from build123d import *

# Parameters (mm, degrees)
F0_R     = 32
F0_W     = 2
F0_H     = 2
F1_DEPTH = 7
F2_R     = 2.5
F4_R     = 2
F5_DEPTH = 7


with BuildPart() as f1:
    # F0 (on Top) → F1 (new body)
    with BuildSketch(Plane.XY):
        Circle(F0_R)
        with BuildLine():
            ThreePointArc((1, 28.9827534924), (20.4757041145, 20.5364442155), (28.9796643011, 1.0858439086))
            Line((28.9796643011, 1.0858439086), (29.9863147924, 1.0858439086))
            Line((29.9863147924, 1.0858439086), (29.9863147924, -0.9141560914))
            Line((29.9863147924, -0.9141560914), (28.9855881196, -0.9141560914))
            ThreePointArc((28.9855881196, -0.9141560914), (20.5364411166, -20.4757072226), (1, -28.9827534924))
            Line((1, -28.9827534924), (1, -29.9833287011))
            Line((1, -29.9833287011), (-1, -29.9833287011))
            Line((-1, -29.9833287011), (-1, -28.9827534924))
            ThreePointArc((-1, -28.9827534924), (-20.5364411166, -20.4757072226), (-28.9855881196, -0.9141560914))
            Line((-28.9855881196, -0.9141560914), (-29.9803426099, -0.9141560914))
            Line((-29.9803426099, -0.9141560914), (-29.9803426099, 1.0858439086))
            Line((-29.9803426099, 1.0858439086), (-28.9796643011, 1.0858439086))
            ThreePointArc((-28.9796643011, 1.0858439086), (-20.4757041145, 20.5364442155), (-1, 28.9827534924))
            Line((-1, 28.9827534924), (-1, 29.9833287011))
            Line((-1, 29.9833287011), (1, 29.9833287011))
            Line((1, 29.9833287011), (1, 28.9827534924))
        make_face(mode=Mode.SUBTRACT)
        with BuildLine():
            ThreePointArc((-1, 28.9827534924), (0, 29), (1, 28.9827534924))
            Line((1, 28.9827534924), (1, 29.9833287011))
            Line((1, 29.9833287011), (-1, 29.9833287011))
            Line((-1, 29.9833287011), (-1, 28.9827534924))
        make_face()
        with BuildLine():
            ThreePointArc((-28.9855881196, -0.9141560914), (-28.9998727937, 0.0858949914), (-28.9796643011, 1.0858439086))
            Line((-28.9796643011, 1.0858439086), (-29.9803426099, 1.0858439086))
            Line((-29.9803426099, 1.0858439086), (-29.9803426099, -0.9141560914))
            Line((-29.9803426099, -0.9141560914), (-28.9855881196, -0.9141560914))
        make_face()
        with BuildLine():
            Line((1, -29.9833287011), (1, -28.9827534924))
            ThreePointArc((1, -28.9827534924), (0, -29), (-1, -28.9827534924))
            Line((-1, -28.9827534924), (-1, -29.9833287011))
            Line((-1, -29.9833287011), (1, -29.9833287011))
        make_face()
        with Locations((0, 0.0858439086)):
            Rectangle(F0_W, F0_H)
        with BuildLine():
            Line((-1, -0.9141560914), (-1, 1.0858439086))
            Line((-1, 1.0858439086), (-28.9796643011, 1.0858439086))
            ThreePointArc((-28.9796643011, 1.0858439086), (-28.9998727937, 0.0858949914), (-28.9855881196, -0.9141560914))
            Line((-28.9855881196, -0.9141560914), (-1, -0.9141560914))
        make_face()
        with BuildLine():
            ThreePointArc((28.9855881196, -0.9141560914), (28.9963968061, -0.4571348438), (29, 0))
            ThreePointArc((29, 0), (28.9949156296, 0.5430171578), (28.9796643011, 1.0858439086))
            Line((28.9796643011, 1.0858439086), (1, 1.0858439086))
            Line((1, 1.0858439086), (1, -0.9141560914))
            Line((1, -0.9141560914), (28.9855881196, -0.9141560914))
        make_face()
        with BuildLine():
            Line((1, 1.0858439086), (1, 28.9827534924))
            ThreePointArc((1, 28.9827534924), (0, 29), (-1, 28.9827534924))
            Line((-1, 28.9827534924), (-1, 1.0858439086))
            Line((-1, 1.0858439086), (1, 1.0858439086))
        make_face()
        with BuildLine():
            ThreePointArc((-1, -28.9827534924), (0, -29), (1, -28.9827534924))
            Line((1, -28.9827534924), (1, -0.9141560914))
            Line((1, -0.9141560914), (-1, -0.9141560914))
            Line((-1, -0.9141560914), (-1, -28.9827534924))
        make_face()
        with BuildLine():
            ThreePointArc((28.9796643011, 1.0858439086), (28.9949156296, 0.5430171578), (29, 0))
            ThreePointArc((29, 0), (28.9963968061, -0.4571348438), (28.9855881196, -0.9141560914))
            Line((28.9855881196, -0.9141560914), (29.9863147924, -0.9141560914))
            Line((29.9863147924, -0.9141560914), (29.9863147924, 1.0858439086))
            Line((29.9863147924, 1.0858439086), (28.9796643011, 1.0858439086))
        make_face()
    extrude(amount=F1_DEPTH)

    # F2 (on Right) → F3 (revolve, cut)
    with BuildSketch(Plane.YZ):
        with Locations((-10, 3.4933774173)):
            Circle(F2_R)
    revolve(axis=Axis((0, 0, 9.8674278706), (0, 0, 1)), mode=Mode.SUBTRACT)

    # F4 (on Top) → F5 (join)
    with BuildSketch(Plane.XY):
        with BuildLine():
            ThreePointArc((5.0092860358, 0.072944447), (6.2053928233, 1.3731565576), (6.6388960149, 3.0858439086))
            ThreePointArc((6.6388960149, 3.0858439086), (4.061145293, 6.5376559564), (0.0194480075, 5.0461841164))
            ThreePointArc((0.0194480075, 5.0461841164), (0.4518120478, 4.1080931867), (0.6, 3.0858439086))
            ThreePointArc((0.6, 3.0858439086), (0.4518120478, 2.0635946305), (0.0194480075, 1.1255037008))
            ThreePointArc((0.0194480075, 1.1255037008), (0.4726534867, 0.5610866358), (1.0296099792, 0.0987433702))
            ThreePointArc((1.0296099792, 0.0987433702), (3.0233371186, 0.685768266), (5.0092860358, 0.072944447))
        make_face()
        with Locations((3.0388960149, 3.0858439086)):
            Circle(F4_R, mode=Mode.SUBTRACT)
        with BuildLine():
            ThreePointArc((6.6, -2.9141560914), (6.1775328266, -1.2220316469), (5.0092860358, 0.072944447))
            ThreePointArc((5.0092860358, 0.072944447), (3.0155588963, -0.5140804488), (1.0296099792, 0.0987433702))
            ThreePointArc((1.0296099792, 0.0987433702), (0.4627203706, -0.360293902), (0, -0.9241812172))
            ThreePointArc((0, -0.9241812172), (0.4467375879, -1.8749256068), (0.6, -2.9141560914))
            ThreePointArc((0.6, -2.9141560914), (0.4467375879, -3.9533865759), (0, -4.9041309656))
            ThreePointArc((0, -4.9041309656), (4.0392304845, -6.3608936793), (6.6, -2.9141560914))
        make_face()
        with Locations((3, -2.9141560914)):
            Circle(F4_R, mode=Mode.SUBTRACT)
        with BuildLine():
            ThreePointArc((-1.0100251258, 0.0858439086), (-3, -0.5141560914), (-4.9899748742, 0.0858439086))
            ThreePointArc((-4.9899748742, 0.0858439086), (-5.5455844123, -5.4597405036), (0, -4.9041309656))
            ThreePointArc((0, -4.9041309656), (-0.6, -2.9141560914), (0, -0.9241812172))
            ThreePointArc((0, -0.9241812172), (-0.4544155877, -0.3685716791), (-1.0100251258, 0.0858439086))
        make_face()
        with Locations((-3, -2.9141560914)):
            Circle(F4_R, mode=Mode.SUBTRACT)
        with BuildLine():
            ThreePointArc((0.0194480075, 1.1255037008), (-0.5611039851, 3.0858439086), (0.0194480075, 5.0461841164))
            ThreePointArc((0.0194480075, 5.0461841164), (-5.5330214127, 5.6439296231), (-4.9899748742, 0.0858439086))
            ThreePointArc((-4.9899748742, 0.0858439086), (-3, 0.6858439086), (-1.0100251258, 0.0858439086))
            ThreePointArc((-1.0100251258, 0.0858439086), (-0.4419142855, 0.5528224959), (0.0194480075, 1.1255037008))
        make_face()
        with Locations((-3, 3.0858439086)):
            Circle(F4_R, mode=Mode.SUBTRACT)
    extrude(amount=F5_DEPTH)


solid = f1.part
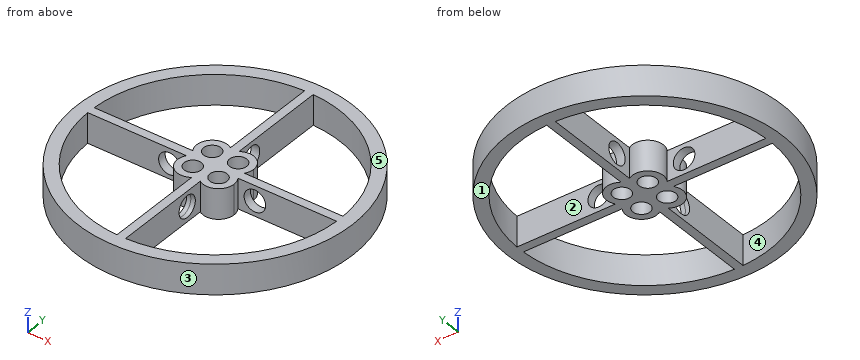
Verification items for the finished model (mm, model axes). Face numbers are marked on the shaded views. A direction names the side the tool comes from. Round coordinates to 2 decimals unless told otherwise and drop trailing zeros. Order: outer loops, then holes, each group sorted by start corner. A loop starts at its lowest first (then second) coordinate and runs counter-clockwise, first axis right, second up. Notation, with made-up numbers: (-8.5, -2) -> (34.5, -2) arc R24 cw to (34.5, 12) -> close; hole circle Ø8 at (54, 52). An arc over 180 degrees is marked (long way). Put each result on its own line as item: value.
1) Section check A-A (x = -22.5). Record the cut outline in (y, z).
Final values:
outline: (-22.75, 0) -> (-18.3, 0) -> (-18.3, 7) -> (-22.75, 7) -> close; (-0.91, 0) -> (1.09, 0) -> (1.09, 7) -> (-0.91, 7) -> close; (18.3, 0) -> (22.75, 0) -> (22.75, 7) -> (18.3, 7) -> close
2) Material ranges on line 1 (X direction, y = -23.5, z = 6); line 2 (Y direction, x = -17.5, z = 4.5); line 3 (X direction, y = 7.5, z = 5.75), recorded low to high.
Final values:
line 1: x = -21.72 to -16.99, -1 to 1, 16.99 to 21.72
line 2: y = -26.79 to -23.12, -0.91 to 1.09, 23.12 to 26.79
line 3: x = -31.11 to -28.01, -1 to 1, 28.01 to 31.11
3) Section check D-D (y = 0). Record the cut outline in (x, z).
Final values:
outline: (-32, 0) -> (32, 0) -> (32, 7) -> (-32, 7) -> close; hole circle Ø5 at (-10, 3.49); hole circle Ø5 at (10, 3.49)
4) Mould release check, pull along X, two halves, no side actions. Record for the marked faces 1, 2 and 3: +X half, -X half, draft (parallel to the pull), parting line (faces both ways), or undercut.
Final values:
face 1: draft
face 2: undercut
face 3: parting line
5) Set-up check for the marked faces 4 and 5: record each of +Z, -Z, +X, -X, +Y, -Y from which the full face is reachable in a straight line by a thin tool's end or side.
Final values:
face 4: +Z, -Z
face 5: +Z, +X, -X, +Y, -Y
6) Depth check by flat-ended pin: pin 1 (3.5 mm diameter, centred on y = -22.5, z = 4.5, fed in from +X); pin 2 (1 mm diameter, centred on x = -18.5, z = 4.5, fed in from -Y); pin 3 (2 mm diameter, centred on x = 15, z = 4.5, fed in from -Y) (3 decimals). Enter the tip coordinate at first touch or a pass-through.
Final values:
pin 1: stops at x = 24.36
pin 2: stops at y = -26.46
pin 3: stops at y = -28.775
7) Section check B-B (y = -21). Record the cut outline in (x, z).
Final values:
outline: (-24.15, 0) -> (-20, 0) -> (-20, 7) -> (-24.15, 7) -> close; (-1, 0) -> (1, 0) -> (1, 7) -> (-1, 7) -> close; (20, 0) -> (24.15, 0) -> (24.15, 7) -> (20, 7) -> close
8) Section check C-C (z = 5.25). Give the number of separate pieces and of enclosed holes in the cut face, then the cut area to 3 significant figures.
Final values:
separate pieces: 2
enclosed holes: 5
area: 835 mm^2
